Design review of the part built by this model. Coordinates are the model's own, in mm. Face numbers are marked on the shaded views. Coordinates: 2 decimals unless noted, no trailing zeros. Write each loop counter-clockwise with the first axis right and the second up, starting at its lowest first coordinate (ties: lowest second). Pieces come first, ordered by that corner, then holes.
Q1. The part is to be moulded in two halves that separate along Z. For the marked faces 1, 2 and 3, say which applies: released by +Z, released by -Z, zero draft, split by the parting line, or undercut.
Q2. For L1, parallel to X at y = -11, z = 14.5; L2, parallel to X at y = -6.5, z = 6.5; L3, parallel to Y at x = -0.5, z = 8.25, list the stretches that pass through material, from the lowest coordinate up.
Q3. Take a section at B-B, the plane y = 0. Write out the cut boundary in (x, z).
Q4. Take a section at C-C, the plane z = 4. Write out the cut boundary in (x, y), plus the area to 3 significant figures.
Q5. For pin 1 Ø4 at (y, z) = (38, 10) entering from +X; pin 2 Ø1.5 at (y, z) = (-6, 3) entering from -X; pin 3 Ø4 at (y, z) = (35, 9) entering from +X, all flat-tipped, find the tip position at first contact; note any pin that passes through.
Q6. Take a section at A-A, the plane x = 0. Write out the cut boundary in (y, z), plus the area to 3 significant figures.
from build123d import *

# Parameters (mm, degrees)
SKETCH_R   = 30
SKETCH_R_2 = 12
PAD_DEPTH  = 16
FILLET_R   = 4


with BuildPart() as part:
    # Sketch → Pad (new body)
    with BuildSketch(Plane.XY):
        with BuildLine():
            ThreePointArc((70.4, -21.629609), (84, 0), (70.4, 21.629609))
            Line((21.666667, 45.061686), (70.4, 21.629609))
            ThreePointArc((21.666667, 45.061686), (0, 50), (-21.666667, 45.061686))
            Line((-70.4, 21.629609), (-21.666667, 45.061686))
            ThreePointArc((-70.4, 21.629609), (-84, 0), (-70.4, -21.629609))
            Line((-21.666667, -45.061686), (-70.4, -21.629609))
            ThreePointArc((-21.666667, -45.061686), (0, -50), (21.666667, -45.061686))
            Line((70.4, -21.629609), (21.666667, -45.061686))
        make_face()
        Circle(SKETCH_R, mode=Mode.SUBTRACT)
        with Locations((60, 0)):
            Circle(SKETCH_R_2, mode=Mode.SUBTRACT)
        with Locations((-60, 0)):
            Circle(SKETCH_R_2, mode=Mode.SUBTRACT)
    extrude(amount=PAD_DEPTH)

    # Fillet
    fillet_edges = [part.edges().sort_by_distance(p)[0] for p in [
        (-46.033333, -33.345648, 16),
        (0, -50, 16),
        (46.033333, -33.345648, 16),
        (84, 0, 16),
        (46.033333, 33.345648, 16),
        (0, 50, 16),
        (-46.033333, 33.345648, 16),
        (-84, 0, 16),
    ]]
    fillet(fillet_edges, radius=FILLET_R)


solid = part.part
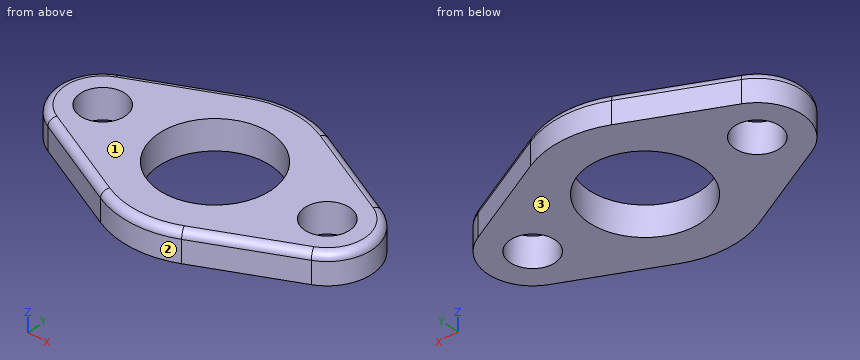
Responses:
1. face 1: released by +Z
1. face 2: zero draft
1. face 3: released by -Z
2. L1: x = -80.34 to -64.8, -55.2 to -27.91, 27.91 to 55.2, 64.8 to 80.34
2. L2: x = -83.1 to -70.09, -49.91 to -29.29, 29.29 to 49.91, 70.09 to 83.1
2. L3: y = -50 to -30, 30 to 50
3. outline: (-84, 0) - (-72, 0) - (-72, 16) - (-80, 16) arc R4 ccw to (-84, 12) - close; (-48, 0) - (-30, 0) - (-30, 16) - (-48, 16) - close; (30, 0) - (48, 0) - (48, 16) - (30, 16) - close; (72, 0) - (84, 0) - (84, 12) arc R4 ccw to (80, 16) - (72, 16) - close
4. outline: (-70.4, -21.63) - (-21.67, -45.06) arc R50 ccw to (21.67, -45.06) - (70.4, -21.63) arc R24 ccw to (70.4, 21.63) - (21.67, 45.06) arc R50 ccw to (-21.67, 45.06) - (-70.4, 21.63) arc R24 ccw to start; hole circle Ø24 at (-60, 0); hole circle Ø60 at (0, 0); hole circle Ø24 at (60, 0)
4. area: 7,800 mm2
5. pin 1: stops at x = 40.51
5. pin 2: stops at x = -83.42
5. pin 3: stops at x = 46.75
6. outline: (-50, 0) - (-30, 0) - (-30, 16) - (-46, 16) arc R4 ccw to (-50, 12) - close; (30, 0) - (50, 0) - (50, 12) arc R4 ccw to (46, 16) - (30, 16) - close
6. area: 633 mm2
